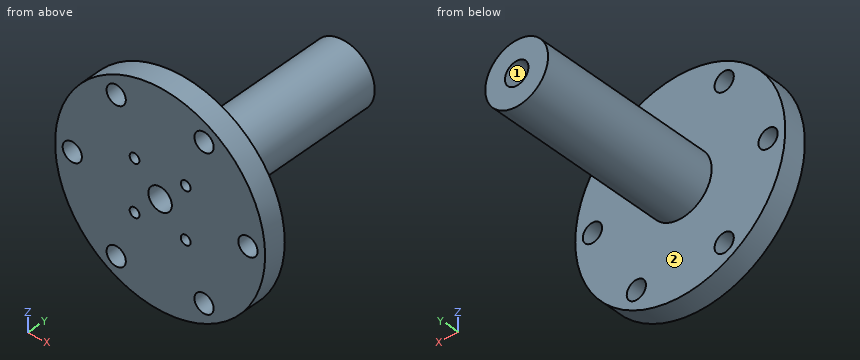
Autodesk Inventor part; units mm, degrees
ref_plane "YZ Plane" through (0, 0, 0) normal (1, 0, 0) x (0, 1, 0)
ref_plane "XZ Plane" through (0, 0, 0) normal (0, 1, 0) x (-1, 0, 0)
ref_plane "XY Plane" through (0, 0, 0) normal (0, 0, 1) x (1, 0, 0)
sketch "Sketch1" plane through (0, 0, 0) normal (0, 0, 1) x (1, 0, 0)
  line L0 (0, 0) -> (0, 26.4) construction
  line L1 (3.175, 56) -> (3.175, 0)
  line L2 (28.4, 0) -> (28.4, 6)
  line L3 (3.175, 0) -> (28.4, 0)
  line L4 (8.5, 56) -> (8.5, 6)
  line L5 (8.5, 6) -> (28.4, 6)
  line L6 (8.5, 56) -> (8.5, -232.68) construction
  line L7 (8.5, 56) -> (8.5, 16.2) construction
  line L8 (8.5, 56) -> (3.175, 56)
  dimension "d0" = 26.4
  dimension "d5" = 6
  dimension "d11" = 5.325
  dimension "d32" = 3.175
  dimension "d37" = 28.4
  dimension "d38" = 50
revolve "Revolution1" add sketch "Sketch1" angle 360 about axis through (0, 0, 0) along (0, 1, 0)
sketch "Sketch4" plane through (0, 6, 0) normal (0, 1, 0) x (1, 0, 0)
  line L0 (0, 0) -> (-23.75, 0) construction
  circle A0 centre (-23.75, 0) radius 2.6
  circle A1 centre (-11.875, -20.5681) radius 2.6
  circle A2 centre (11.875, -20.5681) radius 2.6
  circle A3 centre (23.75, 0) radius 2.6
  circle A4 centre (11.875, 20.5681) radius 2.6
  circle A5 centre (-11.875, 20.5681) radius 2.6
  dimension "d23" = 23.75
  dimension "d24" = 5.2
  dimension "d27" = 360
extrude "Extrusion1" cut sketch "Sketch4" against normal blind 6
sketch "Sketch5" plane through (0, 0, 0) normal (0, -1, 0) x (1, 0, 0)
  circle A0 centre (0, 0) radius 3.175
  line L0 (0, 0) -> (6.9148, -6.9148)
  line L1 (0, 0) -> (9.779, 0) construction
  dimension "d39" = 9.779
  dimension "d40" = 45
hole "Hole2" at (6.9148, 0, -6.9148) direction (0, 1, 0) diameter 2.6416 depth 5.08 tip angle 118
pattern_circular "Circular Pattern1" count 4 over 360 about axis through (0, 28, 0) along (0, -1, 0) of "Hole2"
properties part number "Mechanum Wheel Adapter"
Verification items for the finished model (mm, model axes). Face numbers are marked on the shaded views. A direction names the side the tool comes from. Coordinates: 2 decimals unless noted, no trailing zeros. Order: outer loops, then holes, each group sorted by start corner. A loop starts at its lowest first (then second) coordinate and runs counter-clockwise, first axis right, second up.
Item 1: Material ranges on L1, parallel to X at y = 22, z = 0 (3 decimals); L2, parallel to Y at x = 10, z = -13; L3, parallel to Z at x = 1, y = 48.5, recorded low to high.
Filled in:
L1: x = -8.5 to -3.175, 3.175 to 8.5
L2: y = 0 to 6
L3: z = -8.44 to -3.01, 3.01 to 8.44
Item 2: Section check B-B, the plane z = 0. Enter the section's corners in (x, y) (3 decimals), then the cut area to 3 significant figures.
Filled in:
outline: (-28.4, 0) - (-26.35, 0) - (-26.35, 6) - (-28.4, 6) - close; (-21.15, 0) - (-3.175, 0) - (-3.175, 56) - (-8.5, 56) - (-8.5, 6) - (-21.15, 6) - close; (3.175, 0) - (21.15, 0) - (21.15, 6) - (8.5, 6) - (8.5, 56) - (3.175, 56) - close; (26.35, 0) - (28.4, 0) - (28.4, 6) - (26.35, 6) - close
area: 773 mm2
Item 3: Access from +Z, -Z, +X, -X, +Y, -Y to the whole of each face (thin tool, end or side, straight path). Record for the marked faces 1 and 2.
Filled in:
face 1: +Y, -Y
face 2: +Y
Item 4: Section check D-D, the plane x = 12.5. Enter the section's corners in (y, z).
Filled in:
outline: (0, -25.5) - (6, -25.5) - (6, -23.09) - (0, -23.09) - close; (0, -18.04) - (6, -18.04) - (6, 18.04) - (0, 18.04) - close; (0, 23.09) - (6, 23.09) - (6, 25.5) - (0, 25.5) - close
Item 5: Section check C-C, the plane y = 11.5. Enter the section's corners in (x, z) (3 decimals), then the cut area to 3 significant figures.
Filled in:
outline: circle Ø17 at (0, 0); hole circle Ø6.35 at (0, 0)
area: 195 mm2
Item 6: Section check A-A, the plane x = 0. Enter the section's corners in (y, z) (3 decimals).
Filled in:
outline: (0, -28.4) - (6, -28.4) - (6, -8.5) - (56, -8.5) - (56, -3.175) - (0, -3.175) - close; (0, 3.175) - (56, 3.175) - (56, 8.5) - (6, 8.5) - (6, 28.4) - (0, 28.4) - close
Item 7: Depth check by flat-ended pin: pin 1 (4 mm diameter, centred on x = -11.88, z = 20.57, fed in from -Y); pin 2 (1.6 mm diameter, centred on x = 6.91, z = -6.91, fed in from +Y); pin 3 (10 mm diameter, centred on y = 38, z = 4, fed in from +X); pin 4 (1 mm diameter, centred on x = 0, y = 34.5, fed in from -Z). Enter the tip coordinate at first touch or a pass-through.
Filled in:
pin 1: passes through
pin 2: stops at y = 6
pin 3: stops at x = 8.5
pin 4: stops at z = -8.5
